from build123d import *

# Parameters (mm, degrees)
SKETCH1_R           = 4.5
SKETCH1_R_2         = 1.5
BOSS_EXTRUDE1_DEPTH = 3
BOSS_EXTRUDE2_DEPTH = 7
SKETCH3_R           = 1.5
CUT_EXTRUDE1_DEPTH  = 6.5


with BuildPart() as part:
    # Sketch1 → Boss-Extrude1 (new body)
    with BuildSketch(Plane(origin=(0, 0, 0), x_dir=(1, 0, 0), z_dir=(0, 1, 0))):
        with Locations(Location((0, 0, 0), (0, 0, 270))):
            Circle(SKETCH1_R)
        with Locations(Location((0, 0, 0), (0, 0, 270))):
            Circle(SKETCH1_R_2, mode=Mode.SUBTRACT)
    extrude(amount=BOSS_EXTRUDE1_DEPTH)

    # Sketch2 → Boss-Extrude2 (add)
    with BuildSketch(Plane(origin=(0, 3, 0), x_dir=(1, 0, 0), z_dir=(0, 1, 0))):
        with BuildLine():
            ThreePointArc((-2.9, 3.440930107), (-4.5, 0), (-2.9, -3.440930107))
            Line((-2.9, -3.440930107), (-2.9, 3.440930107))
        make_face()
        with BuildLine():
            Line((2.9, 3.440930107), (2.9, -3.440930107))
            ThreePointArc((2.9, -3.440930107), (4.080441153, -1.897366596), (4.5, 0))
            ThreePointArc((4.5, 0), (4.080441153, 1.897366596), (2.9, 3.440930107))
        make_face()
    extrude(amount=BOSS_EXTRUDE2_DEPTH)

    # Sketch3 → Cut-Extrude1 (cut)
    with BuildSketch(Plane(origin=(-2.9, 0, 0), x_dir=(0, 0, -1), z_dir=(1, 0, 0))):
        with BuildLine():
            Line((2.440930107, 8.984324563), (2.440930107, 3))
            Line((2.440930107, 3), (3.440930107, 3))
            Line((3.440930107, 3), (3.440930107, 10))
            Line((3.440930107, 10), (0, 10))
            ThreePointArc((0, 10), (1.321905479, 9.735949794), (2.440930107, 8.984324563))
        make_face()
        with BuildLine():
            ThreePointArc((-2.440930107, 8.984324563), (-1.321905479, 9.735949794), (0, 10))
            Line((0, 10), (-3.440930107, 10))
            Line((-3.440930107, 10), (-3.440930107, 3))
            Line((-3.440930107, 3), (-2.440930107, 3))
            Line((-2.440930107, 3), (-2.440930107, 8.984324563))
        make_face()
        with Locations((0, 7.7)):
            Circle(SKETCH3_R)
    cut_extrude1 = extrude(amount=-CUT_EXTRUDE1_DEPTH, mode=Mode.SUBTRACT)

    # Mirror1: Cut-Extrude1 across plane
    add(cut_extrude1.mirror(Plane(origin=(0, 0, 0), x_dir=(0, 0, 1), z_dir=(1, 0, 0))), mode=Mode.SUBTRACT)


solid = part.part
The listing builds one solid part. Answer for the finished solid, in the listing's coordinates (mm). A direction names the side the tool comes from. Coordinates: 2 decimals unless noted, no trailing zeros. Loops run counter-clockwise (first coordinate to the right, second up) from the corner with the lowest first, then second, coordinate; pieces in that order, holes last. Notation, with made-up numbers: M -9.75,24.5 L 8.25,24.5 A35 ccw 8.25,57.5 Z; hole C -22.5,-30.75 d4. An arc over 180 degrees is marked long. Answer in a Markdown table with one row per item.
1) Given pin 1 (3 mm diameter, centred on y = 6, z = 2, fed in from -X); pin 2 (1.8 mm diameter, centred on x = 0, z = 0, fed in from +Y); pin 3 (1 mm diameter, centred on x = 3, y = 6.5, fed in from +Z); pin 4 (1.5 mm diameter, centred on x = -1, z = 2, fed in from +Y), each flat-ended and moving along its own axis, determine where each tip first touches the part or whether it passes through.
Answers below:
| item | result |
|---|---|
| pin 1 | x = -4.47 |
| pin 2 | through |
| pin 3 | z = 2.44 |
| pin 4 | y = 3 |
2) Find section D-D (z = 1.25). Determine the outline of the cut face in (x, y), then the cut area to 3 significant figures.
Answers below:
| item | result |
|---|---|
| outline | M -4.32,0 L -0.83,0 L -0.83,3 L -2.9,3 L -2.9,6.87 L -4.32,6.87 Z; M -4.32,8.53 L -2.9,8.53 L -2.9,9.76 L -4.32,9.76 Z; M 0.83,0 L 4.32,0 L 4.32,6.87 L 2.9,6.87 L 2.9,3 L 0.83,3 Z; M 2.9,8.53 L 4.32,8.53 L 4.32,9.76 L 2.9,9.76 Z |
| area | 35.5 mm^2 |
3) Determine the mould class of faces 1 (the cylindrical face through (3.689, 7.125, -1.386)), 2 (the cylindrical face through (0.45, 1.48, 1.43)), 3 (the flat face through (-2, 0, 0)) for opening direction Y: released by +Y, released by -Y, zero draft, split by the parting line, or undercut.
Answers below:
| item | result |
|---|---|
| face 1 | undercut |
| face 2 | zero draft |
| face 3 | released by -Y |
4) Find section B-B (x = 0). Determine the outline of the cut face in (y, z), then the cut area to 3 significant figures.
Answers below:
| item | result |
|---|---|
| outline | M 0,-4.5 L 3,-4.5 L 3,-1.5 L 0,-1.5 Z; M 0,1.5 L 3,1.5 L 3,4.5 L 0,4.5 Z |
| area | 18.0 mm^2 |
5) Which of the six approach directions +Z, -Z, +X, -X, +Y, -Y give full straight-line access (tool end or side, diameter ignored) to faces 4 (the flat face through (-3.3, 6, 2.441)), 5 (the flat face through (3.3, 6, -2.441)), 6 (the flat face through (2.9, 6, 0)), 7 (the cylindrical face through (-3.692, 7.125, -1.386))?
Answers below:
| item | result |
|---|---|
| face 4 | +Z, +X, -X, +Y |
| face 5 | -Z, +X, -X, +Y |
| face 6 | +Z, -Z, +Y |
| face 7 | +X, -X |
6) Find the intervals of material crossed by probe 1 along X at (y, z) = (0.6, 0); probe 2 along Z at (x, y) = (3.3, 7.7); probe 3 along Y at (x, z) = (-3.55, 0), in increasing order.
Answers below:
| item | result |
|---|---|
| probe 1 | -4.5 to -1.5, 1.5 to 4.5 |
| probe 2 | -2.44 to -1.5, 1.5 to 2.44 |
| probe 3 | 0 to 6.2, 9.2 to 10 |
7) Find section A-A (y = 4.5). Determine the outline of the cut face in (x, z).
Answers below:
| item | result |
|---|---|
| outline | M -3.78,-2.44 L -2.9,-2.44 L -2.9,2.44 L -3.78,2.44 A4.5 ccw Z; M 2.9,-2.44 L 3.78,-2.44 A4.5 ccw 3.78,2.44 L 2.9,2.44 Z |
8) Find section C-C (y = 7.7). Determine the outline of the cut face in (x, z).
Answers below:
| item | result |
|---|---|
| outline | M -4.24,-1.5 A4.5 ccw -3.78,-2.44 L -2.9,-2.44 L -2.9,-1.5 Z; M -4.24,1.5 L -2.9,1.5 L -2.9,2.44 L -3.78,2.44 A4.5 ccw Z; M 2.9,-2.44 L 3.78,-2.44 A4.5 ccw 4.24,-1.5 L 2.9,-1.5 Z; M 2.9,1.5 L 4.24,1.5 A4.5 ccw 3.78,2.44 L 2.9,2.44 Z |
